Read the model definition and answer for the solid it produces. Units are mm, in the model's axes. A direction names the side the tool comes from. Give positions to 0.01 mm unless a question says otherwise; leave off trailing zeros. Order: outer loops, then holes, each group sorted by start corner. A loop starts at its lowest first (then second) coordinate and runs counter-clockwise, first axis right, second up.
```python
from build123d import *

# Parameters (mm, degrees)
SKETCH1_W                = 30
SKETCH1_H                = 40
SKETCH1_W_2              = 26
SKETCH1_H_2              = 36
F_20_X_20_X_2_1_DEPTH    = 160.159392621
SKETCH1_ON_SEGMENT_2_W   = 30
SKETCH1_ON_SEGMENT_2_H   = 40
SKETCH1_ON_SEGMENT_2_W_2 = 26
SKETCH1_ON_SEGMENT_2_H_2 = 36
F_20_X_20_X_2_1_2_DEPTH  = 160.159392621
SKETCH_3_R               = 2
CUT_EXTRUDE_1_DEPTH      = 50
SKETCH_4_R               = 2
CUT_EXTRUDE_2_DEPTH      = 50
SKETCH_5_R               = 2
CUT_EXTRUDE_3_DEPTH      = 167.538055882
SKETCH_6_R               = 2
CUT_EXTRUDE_4_DEPTH      = 167.538055882
SKETCH_7_R               = 2
CUT_EXTRUDE_5_DEPTH      = 167.538055882
SKETCH_8_R               = 2
CUT_EXTRUDE_6_DEPTH      = 167.538055882


with BuildPart() as part:
    # Sketch1 → 方形管 20 X 20 X 2(1) (new body)
    with BuildSketch(Plane(origin=(0, -42.556514737, 122.970952591), x_dir=(0, 0.8198063506063987, 0.5726408538564275), z_dir=(0, 0.5726408538564276, -0.8198063506063988))):
        with Locations((-0.273785359, 0)):
            Rectangle(SKETCH1_W, SKETCH1_H)
        with Locations((-0.273785359, 0)):
            Rectangle(SKETCH1_W_2, SKETCH1_H_2, mode=Mode.SUBTRACT)
    extrude(amount=F_20_X_20_X_2_1_DEPTH)

    # 方形管 20 X 20 X 2(1) mitre 1
    split(bisect_by=Plane(origin=(0, 43.339613341, 0), x_dir=(0, -0.966220685, -0.257716099), z_dir=(0, -0.257716099, 0.966220685)), keep=Keep.TOP)


with BuildPart() as body_2:
    # Sketch1 on segment 2 (carried to segment 2) → 20 X 20 X 2_1 2 (new body)
    with BuildSketch(Plane(origin=(0, 44.236616802, 10.11971557), x_dir=(0, 0.996094545, -0.088293021), z_dir=(0, -0.088293021, -0.996094545))):
        with Locations((-0.273785359, 0)):
            Rectangle(SKETCH1_ON_SEGMENT_2_W, SKETCH1_ON_SEGMENT_2_H)
        with Locations((-0.273785359, 0)):
            Rectangle(SKETCH1_ON_SEGMENT_2_W_2, SKETCH1_ON_SEGMENT_2_H_2, mode=Mode.SUBTRACT)
    extrude(amount=F_20_X_20_X_2_1_2_DEPTH)

    # 20 X 20 X 2_1 2 mitre 1
    split(bisect_by=Plane(origin=(0, 43.339613341, 0), x_dir=(0, 0.966220685, 0.257716099), z_dir=(0, 0.257716099, -0.966220685)), keep=Keep.TOP)


with BuildPart() as part_1:
    add(part.part)

    # 方形管 20 X 20 X 2(1) as one body: union body 2
    add(body_2.part)

    # 草图3 → 切除-拉伸1 (cut)
    with BuildSketch(Plane(origin=(0, 41.200437908, 28.778813344), x_dir=(1, 0, 0), z_dir=(0, 0.8198063506064069, 0.5726408538564159))):
        with Locations(Location((-13, -93.181966811, 0), (0, 0, 270))):
            Circle(SKETCH_3_R)
        with Locations(Location((7, -93.181966811, 0), (0, 0, 270))):
            Circle(SKETCH_3_R)
        with Locations(Location((7, -115.181966811, 0), (0, 0, 270))):
            Circle(SKETCH_3_R)
        with Locations(Location((-13, -115.181966811, 0), (0, 0, 270))):
            Circle(SKETCH_3_R)
    extrude(amount=-CUT_EXTRUDE_1_DEPTH, mode=Mode.SUBTRACT)

    # 草图4 → 切除-拉伸2 (cut)
    with BuildSketch(Plane(origin=(0, 57.670454633, -5.111862784), x_dir=(1, 0, 0), z_dir=(0, 0.9960945449749122, -0.08829302051251052))):
        with Locations(Location((-13, 136.17341463, 0), (0, 0, 270))):
            Circle(SKETCH_4_R)
        with Locations(Location((7, 136.17341463, 0), (0, 0, 270))):
            Circle(SKETCH_4_R)
        with Locations(Location((7, 114.17341463, 0), (0, 0, 270))):
            Circle(SKETCH_4_R)
        with Locations(Location((-13, 114.17341463, 0), (0, 0, 270))):
            Circle(SKETCH_4_R)
    extrude(amount=-CUT_EXTRUDE_2_DEPTH, mode=Mode.SUBTRACT)

    # 草图5 → 切除-拉伸3 (cut, through all)
    with BuildSketch(Plane(origin=(20, 0, 0), x_dir=(0, 0, -1), z_dir=(1, 0, 0))):
        with Locations((-88.617234765, -7.915947573)):
            Circle(SKETCH_5_R)
        with Locations((-68.122076, 6.400073774)):
            Circle(SKETCH_5_R)
        with Locations((-58.959822338, -6.716827836)):
            Circle(SKETCH_5_R)
        with Locations((-79.454981103, -21.032849183)):
            Circle(SKETCH_5_R)
    extrude(amount=-CUT_EXTRUDE_3_DEPTH, mode=Mode.SUBTRACT)

    # 草图6 → 切除-拉伸4 (cut, through all)
    with BuildSketch(Plane(origin=(20, 0, 0), x_dir=(0, 0, -1), z_dir=(1, 0, 0))):
        with Locations((-123.00994656, -33.769213815)):
            Circle(SKETCH_6_R)
        with Locations((-96.776143341, -15.444706491)):
            Circle(SKETCH_6_R)
        with Locations((-88.186530533, -27.74180175)):
            Circle(SKETCH_6_R)
        with Locations((-114.420333752, -46.066309074)):
            Circle(SKETCH_6_R)
    extrude(amount=-CUT_EXTRUDE_4_DEPTH, mode=Mode.SUBTRACT)

    # 草图7 → 切除-拉伸5 (cut, through all)
    with BuildSketch(Plane(origin=(20, 0, 0), x_dir=(0, 0, -1), z_dir=(1, 0, 0))):
        with Locations((145.071733339, 37.735118352)):
            Circle(SKETCH_7_R)
        with Locations((143.747338031, 22.793700177)):
            Circle(SKETCH_7_R)
        with Locations((111.872312592, 25.619076833)):
            Circle(SKETCH_7_R)
        with Locations((113.1967079, 40.560495008)):
            Circle(SKETCH_7_R)
    extrude(amount=-CUT_EXTRUDE_5_DEPTH, mode=Mode.SUBTRACT)

    # 草图8 → 切除-拉伸6 (cut, through all)
    with BuildSketch(Plane(origin=(20, 0, 0), x_dir=(0, 0, -1), z_dir=(1, 0, 0))):
        with Locations(Location((-2.502073785, 52.720305714, 0), (0, 0, 284.934586598))):
            Circle(SKETCH_8_R)
        with Locations((7.154223301, 50.121089178)):
            Circle(SKETCH_8_R)
        with Locations((9.731384293, 40.458882327)):
            Circle(SKETCH_8_R)
        with Locations(Location((2.652248199, 33.395892013, 0), (0, 0, 284.934586598))):
            Circle(SKETCH_8_R)
        with Locations((-7.004048886, 35.99510855)):
            Circle(SKETCH_8_R)
        with Locations((-9.581209878, 45.6573154)):
            Circle(SKETCH_8_R)
    extrude(amount=-CUT_EXTRUDE_6_DEPTH, mode=Mode.SUBTRACT)


solid = part_1.part
```
1) Consider L1, parallel to X at y = 44.5, z = -26; L2, parallel to Y at x = 8, z = 43; L3, parallel to Y at x = -5, z = -23.5. Determine where each line is inside the solid, lowest interval first.
Final values:
L1: x = -20 to -18, 18 to 20
L2: y = -5.33 to -2.89, 28.83 to 31.27
L3: y = 25.92 to 27.93, 54.03 to 56.04
2) The part is cut by section A-A on x = 15.5. Determine the outline of the cut face in (y, z), and give its area (3 significant figures).
Final values:
outline: (-55.08, 114.22) - (27.63, -4.19) - (14.88, -148.07) - (16.87, -148.24) - (29.69, -3.64) - (-53.44, 115.37) - close; (-32.12, 130.26) - (56.43, 3.49) - (42.77, -150.54) - (44.76, -150.71) - (58.48, 4.04) - (-30.48, 131.4) - close
area: 1,200 mm2
3) A tool of negligible diameter and unlimited length cuts with its end or side. For faces 4 (the face through (1.57, -53.77, 115.14)), 5 (the face through (-0.252, 23.372, -74.929)), 6 (the face through (-18, 23, 9)), 7 (the face through (-20, 28, -1)), 8 (the face through (-0.28, 21.347, -75.12)), from which of +Z, -Z, +X, -X, +Y, -Y can it reach the whole face along a straight path? Write none if from no direction.
Final values:
face 4: +Z, +X, -X, -Y
face 5: -Z
face 6: none
face 7: +Z, -Z, -X, +Y, -Y
face 8: +X, -X, -Y
4) The part is cut by section C-C on z = 15.5. Determine the outline of the cut face in (x, y).
Final values:
outline: (-20, 13.88) - (20, 13.88) - (20, 50.48) - (-20, 50.48) - close; hole (-18, 16.32) - (18, 16.32) - (18, 48.04) - (-18, 48.04) - close
5) Given pin 1 (5 mm diameter, centred on y = 36, z = 7, fed in from +X); pin 2 (3 mm diameter, centred on x = -0.5, y = 32.5, fed in from -Z); pin 3 (2 mm diameter, centred on x = 4.5, y = -23, fed in from +Z); pin 4 (2 mm diameter, centred on x = -13.5, z = 26.5, fed in from -Y), each flat-ended and moving along its own axis, determine where each tip first touches the part or whether it passes through.
Final values:
pin 1: stops at x = 20
pin 2: stops at z = 35.59
pin 3: stops at z = 122.12
pin 4: stops at y = 5.5
6) For a pull along Z with two mould halves and no side action, classify faces 1 (the face through (18, 23, 9)), 2 (the face through (1.575, 16.472, -148.207)), 3 (the face through (20, 28, -1)) as released by +Z, released by -Z, zero draft, split by the parting line, or undercut.
Final values:
face 1: undercut
face 2: released by -Z
face 3: zero draft
7) The part is cut by section B-B on z = -103. Determine the outline of the cut face in (x, y).
Final values:
outline: (-20, 18.88) - (20, 18.88) - (20, 48.99) - (-20, 48.99) - close; hole (-18, 20.88) - (18, 20.88) - (18, 46.99) - (-18, 46.99) - close
